Read the model definition and answer for the solid it produces. Units are mm, in the model's axes. A direction names the side the tool comes from. Coordinates: 2 decimals unless noted, no trailing zeros. Write each loop counter-clockwise with the first axis right and the second up, starting at its lowest first coordinate (ties: lowest second). Pieces come first, ordered by that corner, then holes.
1) Which of the six approach directions +Z, -Z, +X, -X, +Y, -Y give full straight-line access (tool end or side, diameter ignored) to faces 5 (the face through (0, 12, -5)), 6 (the face through (-3.955, 2.465, -5.158)), 7 (the face through (4.7, 16.9, 2.2))?
2) Determine the mould class of faces 1 (the face through (-0.52, 31.33, -0.04)), 2 (the face through (-0.05, 18.84, 3.99)), 3 (the face through (-6.62, 19.3, 0.04)), 4 (the face through (-4.3, 27.3, -3)) for opening direction X: +X half, -X half, draft (parallel to the pull), parting line (faces both ways), or undercut.
3) The part is cut by section C-C (x = -7.5). Determine the outline of the cut face in (y, z), then the cut area to 3 significant figures.
4) The part is cut by section B-B (y = 12). Determine the outline of the cut face in (x, z), then the cut area to 3 significant figures.
5) Find the intervals of material crossed by line 1 (Y direction, x = 0, z = 1); line 2 (X direction, y = 10.5, z = 0); line 3 (Z direction, x = -8.75, y = 31.5), in increasing order.
6) Each of these flat-tipped pins is pushed along its axis until it touches: pin 1 Ø2 at (x, z) = (-5.5, -0.5) entering from -Y; pin 2 Ø6 at (x, y) = (1.5, 27.5) entering from +Z; pin 3 Ø4 at (x, y) = (-8, 29) entering from -Z; pin 4 Ø5 at (y, z) = (19.5, 0.5) entering from +X. Where does it stop, or does it pass through?
7) The part is cut by section A-A (y = 24). Determine the outline of the cut face in (x, z).
from build123d import *

# Parameters (mm, degrees)
SKETCH1_R           = 6.5
BOSS_EXTRUDE1_DEPTH = 6
FILLET1_R           = 1
SKETCH3_R           = 5
BOSS_EXTRUDE2_DEPTH = 13.83
SKETCH2_R           = 3
CUT_EXTRUDE1_DEPTH  = 15
SKETCH4_R           = 4
BOSS_EXTRUDE4_DEPTH = 3
CHAMFER2_SIZE       = 2


with BuildPart() as part:
    # Sketch1 → Boss-Extrude1 (new body)
    with BuildSketch(Plane(origin=(0, 0, 0), x_dir=(1, 0, 0), z_dir=(0, 1, 0))):
        with Locations(Location((0, 0, 0), (0, 0, 270))):
            Circle(SKETCH1_R)
    extrude(amount=BOSS_EXTRUDE1_DEPTH)

    # Fillet1
    fillet1_edges = [part.edges().sort_by_distance(p)[0] for p in [
        (0, 6, -6.5),
    ]]
    fillet(fillet1_edges, radius=FILLET1_R)

    # Sketch3 → Boss-Extrude2 (add)
    with BuildSketch(Plane(origin=(0, 6, 0), x_dir=(1, 0, 0), z_dir=(0, 1, 0))):
        with Locations(Location((0, 0, 0), (0, 0, 270))):
            Circle(SKETCH3_R)
    extrude(amount=BOSS_EXTRUDE2_DEPTH)

    # Sketch2 → Cut-Extrude1 (cut)
    with BuildSketch(Plane.XZ):
        with Locations(Location((0, 0, 0), (0, 0, 270))):
            Circle(SKETCH2_R)
    extrude(amount=-CUT_EXTRUDE1_DEPTH, mode=Mode.SUBTRACT)

    # Sketch4 → Boss-Extrude4 (add, symmetric)
    with BuildSketch(Plane.XY):
        with BuildLine():
            Line((-5, 16.9), (-8.286276315, 21.764413101))
            ThreePointArc((-8.286276315, 21.764413101), (0, 37.362414962), (8.286276315, 21.764413101))
            Line((8.286276315, 21.764413101), (5, 16.9))
            Line((5, 16.9), (-5, 16.9))
        make_face()
        with Locations((0, 27.362414962)):
            Circle(SKETCH4_R, mode=Mode.SUBTRACT)
    extrude(amount=BOSS_EXTRUDE4_DEPTH, both=True)

    # Chamfer2
    chamfer2_edges = [part.edges().sort_by_distance(p)[0] for p in [
        (0, 19.83, -5),
        (2.236067977, 19.83, 4.472135955),
    ]]
    chamfer(chamfer2_edges, length=CHAMFER2_SIZE - 0.0001)  # a hair under: the kernel refuses the full size


solid = part.part
Reported:
1. face 5: none
1. face 6: -Y
1. face 7: +Z, +X
2. face 1: undercut
2. face 2: parting line
2. face 3: -X half
2. face 4: draft
3. outline: (20.6, -3) - (33.98, -3) - (33.98, 3) - (20.6, 3) - close
3. area: 80.3 mm2
4. outline: circle Ø10 at (0, 0); hole circle Ø6 at (0, 0)
4. area: 50.3 mm2
5. line 1: y = 15 to 23.36, 31.36 to 37.36
5. line 2: x = -5 to -3, 3 to 5
5. line 3: z = -3 to 3
6. pin 1: stops at y = 0
6. pin 2: stops at z = 3
6. pin 3: stops at z = -3
6. pin 4: stops at x = 8.44
7. outline: (-9.42, -3) - (-2.17, -3) - (-2.17, 3) - (-9.42, 3) - close; (2.17, -3) - (9.42, -3) - (9.42, 3) - (2.17, 3) - close
